```python
from build123d import *

# Parameters (mm, degrees)
SKETCH1_R           = 60
SKETCH1_R_2         = 4.25
BOSS_EXTRUDE1_DEPTH = 5
SERVO_HOUSING_DEPTH = 27.5
SKETCH4_R           = 2.155
CUT_EXTRUDE1_DEPTH  = 6
SKETCH5_R           = 15
SKETCH5_R_2         = 4.25
BOSS_EXTRUDE2_DEPTH = 49
BEARING_CUT_R       = 11.11
CUT_EXTRUDE2_DEPTH  = 18
CUT_EXTRUDE3_START  = -9
SKETCH6_R           = 11.11
CUT_EXTRUDE3_DEPTH  = 9
SKETCH8_R           = 12.5
CUT_EXTRUDE4_DEPTH  = 10
FILLET1_R           = 2
FILLET2_R           = 2
FILLET5_R           = 2
SKETCH9_R           = 2.5
CUT_EXTRUDE5_DEPTH  = 10


with BuildPart() as part:
    # Sketch1 → Boss-Extrude1 (new body)
    with BuildSketch(Plane(origin=(0, 0, 0), x_dir=(1, 0, 0), z_dir=(0, 1, 0))):
        with Locations(Location((0, 0, 0), (0, 0, 270))):
            Circle(SKETCH1_R)
        with Locations(Location((0, 0, 0), (0, 0, 270))):
            Circle(SKETCH1_R_2, mode=Mode.SUBTRACT)
    extrude(amount=BOSS_EXTRUDE1_DEPTH)

    # Sketch2 → Servo housing (add)
    with BuildSketch(Plane(origin=(0, 5, 0), x_dir=(1, 0, 0), z_dir=(0, 1, 0))):
        Polygon((19.5, 10.5), (27.5, 10.5), (27.5, 18.5), (19.5, 18.5), (14.5, 15.5), (14.5, -35.5), (19.5, -38.5), (40.5, -38.5), (45.5, -35.5), (45.5, 15.5), (40.5, 18.5), (32.5, 18.5), (32.5, 10.5), (40.5, 10.5), (40.5, -30.5), (19.5, -30.5), align=None)
    extrude(amount=SERVO_HOUSING_DEPTH)

    # Sketch4 → Cut-Extrude1 (cut)
    with BuildSketch(Plane(origin=(0, 32.5, 0), x_dir=(1, 0, 0), z_dir=(0, 1, 0))):
        with Locations(Location((25, -34, 0), (0, 0, 270))):
            Circle(SKETCH4_R)
        with Locations(Location((25, 14, 0), (0, 0, 270))):
            Circle(SKETCH4_R)
        with Locations(Location((35, -34, 0), (0, 0, 90))):
            Circle(SKETCH4_R)
        with Locations(Location((35, 14, 0), (0, 0, 90))):
            Circle(SKETCH4_R)
    extrude(amount=-CUT_EXTRUDE1_DEPTH, mode=Mode.SUBTRACT)

    # Sketch5 → Boss-Extrude2 (add)
    with BuildSketch(Plane(origin=(0, 5, 0), x_dir=(1, 0, 0), z_dir=(0, 1, 0))):
        with Locations(Location((0, 0, 0), (0, 0, 14.835111582))):
            Circle(SKETCH5_R)
        with Locations(Location((0, 0, 0), (0, 0, 270))):
            Circle(SKETCH5_R_2, mode=Mode.SUBTRACT)
    extrude(amount=BOSS_EXTRUDE2_DEPTH)

    # Bearing cut → Cut-Extrude2 (cut)
    with BuildSketch(Plane.XZ):
        with Locations(Location((0, 0, 0), (0, 0, 270))):
            Circle(BEARING_CUT_R)
    extrude(amount=-CUT_EXTRUDE2_DEPTH, mode=Mode.SUBTRACT)

    # Sketch6 → Cut-Extrude3 (cut)
    with BuildSketch(Plane(origin=(0, 54, 0), x_dir=(1, 0, 0), z_dir=(0, 1, 0)).offset(CUT_EXTRUDE3_START)):
        with Locations(Location((0, 0, 0), (0, 0, 90))):
            Circle(SKETCH6_R)
    extrude(amount=CUT_EXTRUDE3_DEPTH, mode=Mode.SUBTRACT)

    # Sketch8 → Cut-Extrude4 (cut)
    with BuildSketch(Plane(origin=(0, 0, 0), x_dir=(-1, 0, 0), z_dir=(0, -1, 0))):
        with Locations(Location((0, 0, 0), (0, 0, 90))):
            Circle(SKETCH8_R)
    extrude(amount=-CUT_EXTRUDE4_DEPTH, mode=Mode.SUBTRACT)

    # Fillet1
    fillet1_edges = [part.edges().sort_by_distance(p)[0] for p in [
        (27.5, 18.75, -10.5),
        (32.5, 18.75, -10.5),
    ]]
    fillet(fillet1_edges, radius=FILLET1_R)

    # Fillet2
    fillet2_edges = [part.edges().sort_by_distance(p)[0] for p in [
        (27.5, 18.75, -18.5),
        (19.5, 18.75, -18.5),
        (14.5, 18.75, -15.5),
        (14.5, 18.75, 35.5),
        (19.5, 18.75, 38.5),
        (40.5, 18.75, 38.5),
        (45.5, 18.75, 35.5),
        (45.5, 18.75, -15.5),
        (40.5, 18.75, -18.5),
        (32.5, 18.75, -18.5),
    ]]
    fillet(fillet2_edges, radius=FILLET2_R)

    # Fillet5
    fillet5_edges = [part.edges().sort_by_distance(p)[0] for p in [
        (-14.5, 54, 3.840572874),
    ]]
    fillet(fillet5_edges, radius=FILLET5_R)

    # Sketch9 → Cut-Extrude5 (cut)
    with BuildSketch(Plane.XZ):
        with Locations(Location((0.712812299, 50, 0), (0, 0, 270))):
            Circle(SKETCH9_R)
        with Locations(Location((42.94486404, -25.617313559, 0), (0, 0, 270))):
            Circle(SKETCH9_R)
        with Locations(Location((-43.657676339, -24.382686441, 0), (0, 0, 270))):
            Circle(SKETCH9_R)
    extrude(amount=-CUT_EXTRUDE5_DEPTH, mode=Mode.SUBTRACT)


solid = part.part
```
Could you check a few things on this model? Use its own coordinates, in mm. A direction names the side the tool comes from. Give positions to 0.01 mm unless a question says otherwise; leave off trailing zeros. Order: outer loops, then holes, each group sorted by start corner. A loop starts at its lowest first (then second) coordinate and runs counter-clockwise, first axis right, second up.
Q1. Suppose I cut it at C-C, the plane z = 50. Write out the boundary of the cut face in (x, y).
Q2. For faces 4 (the flat face through (37, 19, -18.5)), 5 (the cylindrical face through (-10.846, 13.944, 2.408)), 6 (the flat face through (43, 19, 37)), 7 (the flat face through (19.5, 19, 10)), which set-ups out of +Z, -Z, +X, -X, +Y, -Y let a thin tool reach every point of the face, with its end or its side?
Q3. I'm going to push flat-ended pins straight in: P1, Ø2, axis at x = -9.5, y = 45.5, coming from the -Z side; P2, Ø5.5, axis at x = 25, z = 34, coming from the +Y side; P3, Ø4, axis at y = 45, z = 9, coming from the +X side; P4, Ø4.5, axis at x = 0.71, z = 50, coming from the +Y side (1 decimal). Where does each tip first touch, or does it pass through?
Q4. If I drill on line 1 along X through (y, z) = (7, 0); line 2 along Z through (x, y) = (40, 6.5); line 3 along X through (y, z) = (15, 12), over which ranges is the centre line in solid material (lowest first)?
Q5. We'd pull the mould along X, two halves only. Please class faces 1 (the flat face through (8, 54, -8)), 2 (the cylindrical face through (2.64, 2.46, -59.94)), 3 (the flat face through (25, 26.5, -14)): +X half, -X half, draft (parallel to the pull), parting line (faces both ways), or undercut.
Solution:
1. outline: (-33.17, 0) - (-1.79, 0) - (-1.79, 5) - (-33.17, 5) - close; (3.21, 0) - (33.17, 0) - (33.17, 5) - (3.21, 5) - close
2. face 4: -Z, +X, -X, +Y
2. face 5: -Y
2. face 6: +Z, +X, +Y
2. face 7: +Y
3. P1: stops at z = -12.36
3. P2: stops at y = 32.5
3. P3: stops at x = 13.27
3. P4: passes through
4. line 1: x = -15 to -12.5, 12.5 to 19.5, 40.5 to 45.5
4. line 2: z = -18.5 to -10.5, 30.5 to 38.5
4. line 3: x = -9 to 9, 14.5 to 19.5, 40.5 to 45.5
5. face 1: draft
5. face 2: parting line
5. face 3: undercut
